from build123d import *

# Parameters (mm, degrees)
SKETCH_1_R      = 2
SKETCH_1_R_2    = 25
SKETCH_1_R_3    = 2.05
SKETCH_1_R_4    = 2.55
SKETCH_1_W      = 8.1
SKETCH_1_H      = 4.13
SKETCH_1_W_2    = 8.2
SKETCH_1_H_2    = 2.1
EXTRUDE_1_DEPTH = 2
FILLET_2_R      = 2


with BuildPart() as part:
    # 草图1 → 凸台-拉伸1 (new body)
    with BuildSketch(Plane.XY):
        Polygon((7.045333707, -5.153917555), (20.793199876, -17.15268299), (73.209787659, -17.315490317), (86.900465187, -17.315490317), (86.900465187, 75.181701178), (67.533287282, 94.548879082), (64.033108715, 91.048700515), (62.548184475, 89.563776275), (56.749908869, 95.362051881), (58.234833109, 96.846976121), (61.771734574, 100.31043179), (54.027552903, 108.054613461), (46.320094131, 115.762072234), (42.819915564, 112.261893667), (41.334991323, 110.776969426), (35.536715718, 116.575245032), (37.021639958, 118.060169273), (40.521818525, 121.560347839), (21.15464062, 140.927525744), (-114.884210676, 140.927525744), (-121.955278488, 123.856457932), (-100.778610768, 102.679790212), (-97.299097838, 106.179996932), (-95.818582675, 107.669317198), (-90.003141638, 101.888257991), (-91.483656801, 100.398937726), (-94.97172112, 96.890128759), (-87.254003865, 89.218039899), (-79.525883533, 81.535609468), (-76.073106039, 84.988386963), (-74.583785773, 86.468902126), (-68.802726567, 80.653461089), (-70.292046832, 79.172945926), (-73.790498852, 75.674493907), (-21.601590364, 23.48558542), (-18.103138345, 26.984037439), (-16.622623182, 28.473357705), (-10.807182146, 22.692298498), (-12.287697308, 21.202978233), (-15.740474803, 17.750200738), (-8.058044372, 10.022080406), (-0.385955513, 2.304363151), (3.122853454, 5.79242747), (4.61217372, 7.272942633), (10.393232926, 1.457501596), (8.903912661, -0.023013566), (5.403705941, -3.502526497), align=None)
        with Locations((-52.972571837, 134.927525744)):
            Circle(SKETCH_1_R, mode=Mode.SUBTRACT)
        with Locations((47.027428163, 14.927525744)):
            Circle(SKETCH_1_R_2, mode=Mode.SUBTRACT)
        with Locations(Location((-22.972571837, 134.927525744, 0), (0, 0, 180))):
            Circle(SKETCH_1_R, mode=Mode.SUBTRACT)
        with Locations((7.027428163, 134.927525744)):
            Circle(SKETCH_1_R, mode=Mode.SUBTRACT)
        with Locations(Location((-112.972571837, 134.927525744, 0), (0, 0, 180))):
            Circle(SKETCH_1_R, mode=Mode.SUBTRACT)
        with Locations((-82.972571837, 134.927525744)):
            Circle(SKETCH_1_R, mode=Mode.SUBTRACT)
        with Locations((49.784912216, 103.811972774)):
            Circle(SKETCH_1_R, mode=Mode.SUBTRACT)
        with Locations((-83.04451802, 93.427525744)):
            Circle(SKETCH_1_R, mode=Mode.SUBTRACT)
        with Locations((20.275835807, 56.927525744)):
            Circle(SKETCH_1_R_3, mode=Mode.SUBTRACT)
        with Locations((70.527428163, -8.572474256)):
            Circle(SKETCH_1_R_4, mode=Mode.SUBTRACT)
        with Locations((23.400215706, -8.445261799)):
            Circle(SKETCH_1_R_4, mode=Mode.SUBTRACT)
        with Locations((23.527428163, 38.681950658)):
            Circle(SKETCH_1_R_4, mode=Mode.SUBTRACT)
        with Locations((70.65464062, 38.554738201)):
            Circle(SKETCH_1_R_4, mode=Mode.SUBTRACT)
        with Locations((6.845259268, 78.01353091)):
            Circle(SKETCH_1_R_3, mode=Mode.SUBTRACT)
        with Locations(Location((-3.848558527, 14.231566251, 0), (0, 0, 180))):
            Circle(SKETCH_1_R, mode=Mode.SUBTRACT)
        with Locations((-6.58531727, 105.099536075)):
            Circle(SKETCH_1_R_3, mode=Mode.SUBTRACT)
        with Locations((-37.972571837, 134.927525744)):
            Rectangle(SKETCH_1_W, SKETCH_1_H, mode=Mode.SUBTRACT)
        with Locations((-7.972571837, 134.927525744)):
            Rectangle(SKETCH_1_W, SKETCH_1_H, mode=Mode.SUBTRACT)
        with Locations((-97.972571837, 134.927525744)):
            Rectangle(SKETCH_1_W, SKETCH_1_H, mode=Mode.SUBTRACT)
        with Locations((-67.972571837, 134.927525744)):
            Rectangle(SKETCH_1_W, SKETCH_1_H, mode=Mode.SUBTRACT)
        with Locations((5.275835807, 56.927525744)):
            Rectangle(SKETCH_1_W_2, SKETCH_1_H_2, mode=Mode.SUBTRACT)
        with Locations((35.275835807, 56.927525744)):
            Rectangle(SKETCH_1_W_2, SKETCH_1_H_2, mode=Mode.SUBTRACT)
        Polygon((-26.317798475, 106.178700743), (-58.783300448, 90.379511607), (-82.786741677, 114.382952836), (-76.96930946, 119.927525744), (-32.606331473, 119.927525744), align=None, mode=Mode.SUBTRACT)
        Polygon((47.310357667, 85.180238498), (24.91351613, 73.844882053), (4.862626833, 105.32477825), (-2.731253041, 121.927525744), (2.38765218, 121.927525744), align=None, mode=Mode.SUBTRACT)
        Polygon((-14.950211349, 60.812452014), (-17.845757969, 76.937806676), (-38.27290612, 66.997027771), (-24.925284185, 50.558567838), align=None, mode=Mode.SUBTRACT)
        Polygon((2.01437662, 34.262984309), (13.802642778, 20.368597473), (13.802642778, 31.617034086), align=None, mode=Mode.SUBTRACT)
    extrude(amount=EXTRUDE_1_DEPTH)

    # 圆角2
    fillet_2_edges = [part.edges().sort_by_distance(p)[0] for p in [
        (-26.317798475, 106.178700743, 1),
        (-32.606331473, 119.927525744, 1),
        (-76.96930946, 119.927525744, 1),
        (-82.786741677, 114.382952836, 1),
        (-58.783300448, 90.379511607, 1),
        (47.310357667, 85.180238498, 1),
        (2.38765218, 121.927525744, 1),
        (-2.731253041, 121.927525744, 1),
        (24.91351613, 73.844882053, 1),
        (-24.925284185, 50.558567838, 1),
        (-14.950211349, 60.812452014, 1),
        (-17.845757969, 76.937806676, 1),
        (-38.27290612, 66.997027771, 1),
        (13.802642778, 31.617034086, 1),
        (2.01437662, 34.262984309, 1),
        (13.802642778, 20.368597473, 1),
        (40.521818525, 121.560347839, 1),
        (46.320094131, 115.762072234, 1),
        (61.771734574, 100.31043179, 1),
        (67.533287282, 94.548879082, 1),
        (86.900465187, -17.315490317, 1),
        (5.403705941, -3.502526497, 1),
        (-0.385955513, 2.304363151, 1),
        (-21.601590364, 23.48558542, 1),
        (-79.525883533, 81.535609468, 1),
        (-94.97172112, 96.890128759, 1),
        (-100.778610768, 102.679790212, 1),
        (-121.955278488, 123.856457932, 1),
        (-114.884210676, 140.927525744, 1),
    ]]
    fillet(fillet_2_edges, radius=FILLET_2_R)


solid = part.part
For this review, take the finished solid that the model builds, in its own axes (mm). Coordinates: 2 decimals unless noted, no trailing zeros. Loops run counter-clockwise (first coordinate to the right, second up) from the corner with the lowest first, then second, coordinate; pieces in that order, holes last. Notation, with made-up numbers: (-17.5, -7) - (2.5, -7) arc R21 cw to (2.5, 6) - close; hole circle Ø2 at (68, 67.25). An arc over 180 degrees is marked (long way). Use a Markdown table: item, result. Add a question column.
Item 1: For line 1 (Y direction, x = 69, z = 0.5); line 2 (X direction, y = 102.5, z = 1.1); line 3 (X direction, y = 75, z = 1.5), list the stretches that pass through material, from the lowest coordinate up.
Item 2: We need section A-A (z = 1.45). Give the number of separate pieces and of enclosed holes in the cut face, and give its area (3 significant figures).
Item 3: We need section B-B (x = -106.5). Give the boundary of the cut face in (y, z).
Item 4: Mouldability with a two-part tool opening along X and no side actions: class faces 1 (the face through (-52.05, 133.153, 0.986)), 2 (the face through (38.476, 113.636, 0.986)), 3 (the face through (13.823, -11.069, 0.986)), 4 (the face through (30.257, 131.825, 0.986)) as pulls with the +X half, pulls with the -X half, needs draft (parallel to the pull), parting line crosses it, or undercut.
Item 5: Insertion check: pin 1 Ø1 at (y, z) = (113.5, 1.5) entering from -X; pin 2 Ø1 at (x, z) = (45, 1.5) entering from -Y; pin 3 Ø1 at (y, z) = (135.5, 1) entering from -X. Each pin has a flat end and moves straight along its axis. Give the tip position at first contact, or say it passes through.
Results list:
| question | item | result |
|---|---|---|
| 1 | line 1 | y = -17.3 to -10.61, -6.53 to 3, 26.85 to 36.61, 40.5 to 93.08 |
| 1 | line 2 | x = -90.62 to -70.9, -33.88 to 6.66, 26.14 to 48.28, 51.29 to 59.58 |
| 1 | line 3 | x = -73.12 to -21.83, -17.63 to 24.25, 27.2 to 86.9 |
| 2 | separate pieces | 1 |
| 2 | enclosed holes | 26 |
| 2 | area | 15,900 mm^2 |
| 3 | outline | (108.4, 0) - (140.93, 0) - (140.93, 2) - (108.4, 2) - close |
| 4 | face 1 | undercut |
| 4 | face 2 | undercut |
| 4 | face 3 | pulls with the -X half |
| 4 | face 4 | pulls with the +X half |
| 5 | pin 1 | stops at x = -112.1 |
| 5 | pin 2 | stops at y = -17.23 |
| 5 | pin 3 | stops at x = -117.34 |
